Source: CAD feature listing. Evaluate the final solid. Frame: model axes, mm. A direction names the side the tool comes from. Give positions to 0.01 mm unless a question says otherwise; leave off trailing zeros. Write each loop counter-clockwise with the first axis right and the second up, starting at its lowest first coordinate (ties: lowest second). Pieces come first, ordered by that corner, then holes. Notation, with made-up numbers: (-36, 86.5) -> (20, 86.5) arc R18 cw to (20, 105.5) -> close; hole circle Ø9 at (32, 79). An arc over 180 degrees is marked (long way). Use one line per item in the form item = value. Start each with the question number.
(1) Cut plane B-B, the plane z = -10. Output: boundary loops of the cut face in (x, y), and give its area (3 significant figures).
(2) Set-up query: faces 1 (the face through (92, 2, -15)), 2 (the face through (53.09, 2.46, -52.77)). Return all of +Z, -Z, +X, -X, +Y, -Y with unobstructed straight access to the full face (end or side cutting, diameter ignored); none if empty.
(3) Draft query along X for faces 3 (the face through (28.45, 2.46, -9.19)), 4 (the face through (60, 2, -60)), 5 (the face through (30.08, 2.46, -71.75)), 6 (the face through (36, 0, -35)). Return one class per face: pulls with the +X half, pulls with the -X half, needs draft (parallel to the pull), parting line crosses it, or undercut.
(4) Cut plane A-A, the plane x = 10. Output: boundary loops of the cut face in (y, z), and give its area (3 significant figures).
(5) Cut plane C-C, the plane y = 1. Count the separate pieces of the cut face and the enclosed holes in it, and give its area (3 significant figures).
(6) Cut plane D-D, the plane z = -88.6. Output: boundary loops of the cut face in (x, y), and give its area (3 significant figures).
(7) Material intervals for line 1 along X through (y, z) = (1.4, -10); line 2 along Z through (x, y) = (31.5, 0.55); line 3 along Z through (x, y) = (43, 1.8), sorted ascending. Write a range as from..to.
(8) First-contact query: P1, Ø2, axis at x = 10, z = -30, coming from the -Y side; P2, Ø4, axis at x = 10, z = -10, coming from the +Y side; P3, Ø2, axis at x = 53, y = 2, coming from the -Z side; P4, Ø3, axis at y = 2.5, z = -54, coming from the +X side. Flat tips, straight axial feed; report the tip coordinate or a pass-through.
from build123d import *

# Parameters (mm, degrees)
ESBO_O1_R                  = 1.75
RESSALTO_EXTRUS_O1_DEPTH   = 5
RESSALTO_EXTRUS_O3_DEPTH   = 5
CORTE_EXTRUS_O1_DEPTH      = 131.203684057
CORTE_EXTRUS_O1_DEPTH_BACK = 131.203684057
ESBO_O3_R                  = 1.5
FILETE1_R                  = 5


with BuildPart() as part:
    # Esboço1 → Ressalto-extrusão1 (new body)
    with BuildSketch(Plane(origin=(0, 0, 0), x_dir=(1, 0, 0), z_dir=(0, 1, 0))):
        Polygon((0, 79.999998212), (0, 0), (79.999998212, 0), (79.999998212, 39.999999106), (39.999999106, 79.999998212), align=None)
        with Locations(Location((10, 69.999998212, 0), (0, 0, 270))):
            Circle(ESBO_O1_R, mode=Mode.SUBTRACT)
        with Locations(Location((30, 69.999998212, 0), (0, 0, 270))):
            Circle(ESBO_O1_R, mode=Mode.SUBTRACT)
        with Locations(Location((10, 29.999998212, 0), (0, 0, 270))):
            Circle(ESBO_O1_R, mode=Mode.SUBTRACT)
        with Locations(Location((69.999998212, 30, 0), (0, 0, 270))):
            Circle(ESBO_O1_R, mode=Mode.SUBTRACT)
        with Locations(Location((29.999998212, 10, 0), (0, 0, 270))):
            Circle(ESBO_O1_R, mode=Mode.SUBTRACT)
        with Locations(Location((69.999998212, 10, 0), (0, 0, 270))):
            Circle(ESBO_O1_R, mode=Mode.SUBTRACT)
        with BuildLine():
            Line((40, 63.443648132), (40, 41))
            ThreePointArc((40, 41), (40.292893219, 40.292893219), (41, 40))
            Line((41, 40), (63.443648132, 40))
            ThreePointArc((63.443648132, 40), (64.367527664, 40.617316568), (64.150754913, 41.707106781))
            Line((64.150754913, 41.707106781), (41.707106781, 64.150754913))
            ThreePointArc((41.707106781, 64.150754913), (40.617316568, 64.367527664), (40, 63.443648132))
        make_face(mode=Mode.SUBTRACT)
    extrude(amount=RESSALTO_EXTRUS_O1_DEPTH)

    # Esboço5 → Ressalto-extrusão3 (add)
    with BuildSketch(Plane.XZ):
        Polygon((79.999998212, 0), (91.999998212, 0), (91.999998212, -27.999999106), (79.999998212, -39.999999106), align=None)
        Polygon((39.999999106, -79.999998212), (27.999999106, -91.999998212), (0, -91.999998212), (0, -79.999998212), align=None)
    extrude(amount=-RESSALTO_EXTRUS_O3_DEPTH)

    # Esboço3 → Corte-extrusão1 (cut, two sides: drawn at the far end of the back side and taken through both)
    with BuildSketch(Plane.XZ.offset(-CORTE_EXTRUS_O1_DEPTH_BACK)):
        with Locations(Location((42.3, -10, 0), (0, 0, 270))):
            Circle(ESBO_O3_R)
        with Locations(Location((10, -88.6, 0), (0, 0, 270))):
            Circle(ESBO_O3_R)
        with Locations(Location((10, -10, 0), (0, 0, 270))):
            Circle(ESBO_O3_R)
    extrude(amount=CORTE_EXTRUS_O1_DEPTH + CORTE_EXTRUS_O1_DEPTH_BACK, mode=Mode.SUBTRACT)

    # Filete1
    filete1_edges = [part.edges().sort_by_distance(p)[0] for p in [
        (91.999998212, 2.5, -27.999999106),
        (91.999998212, 2.5, 0),
        (0, 2.5, -91.999998212),
        (27.999999106, 2.5, -91.999998212),
        (0, 2.5, 0),
    ]]
    fillet(filete1_edges, radius=FILETE1_R)


solid = part.part
Geometry says:
q1.outline = (0, 0) -> (8.5, 0) -> (8.5, 5) -> (0, 5) -> close; (11.5, 0) -> (28.25, 0) -> (28.25, 5) -> (11.5, 5) -> close; (31.75, 0) -> (40.8, 0) -> (40.8, 5) -> (31.75, 5) -> close; (43.8, 0) -> (68.25, 0) -> (68.25, 5) -> (43.8, 5) -> close; (71.75, 0) -> (92, 0) -> (92, 5) -> (71.75, 5) -> close
q1.area = 395 mm^2
q2.face_1 = +Z, -Z, +X, +Y, -Y
q2.face_2 = +Y, -Y
q3.face_3 = undercut
q3.face_4 = pulls with the +X half
q3.face_5 = undercut
q3.face_6 = needs draft
q4.outline = (0, -92) -> (5, -92) -> (5, -90.1) -> (0, -90.1) -> close; (0, -87.1) -> (5, -87.1) -> (5, -71.75) -> (0, -71.75) -> close; (0, -68.25) -> (5, -68.25) -> (5, -31.75) -> (0, -31.75) -> close; (0, -28.25) -> (5, -28.25) -> (5, -11.5) -> (0, -11.5) -> close; (0, -8.5) -> (5, -8.5) -> (5, 0) -> (0, 0) -> close
q4.area = 395 mm^2
q5.separate_pieces = 1
q5.enclosed_holes = 10
q5.area = 5,990 mm^2
q6.outline = (0.26, 0) -> (8.5, 0) -> (8.5, 5) -> (0.26, 5) -> close; (11.5, 0) -> (31.4, 0) -> (31.4, 5) -> (11.5, 5) -> close
q6.area = 141 mm^2
q7.line_1 = 0..8.5, 11.5..28.25, 31.75..40.8, 43.8..68.25, 71.75..92
q7.line_2 = -88.5..-70.9, -69.1..-10.9, -9.1..0
q7.line_3 = -77..-62.86, -40..-11.33, -8.67..0
q8.P1 = through
q8.P2 = 5
q8.P3 = -68
q8.P4 = 67.5
